Work out the finished part from the listing and answer in its coordinate system (mm). Face numbers are marked on the shaded views. A direction names the side the tool comes from. Give positions to 0.01 mm unless a question says otherwise; leave off trailing zeros. Loops run counter-clockwise (first coordinate to the right, second up) from the corner with the lowest first, then second, coordinate; pieces in that order, holes last. Notation, with made-up numbers: M -27,-36 L -8,-36 A23 ccw -8,-9 Z; hole C 64.5,23.25 d2. An arc over 180 degrees is marked long. Use a Markdown table: item, result.
```python
from build123d import *

# Parameters (mm, degrees)
F1_DEPTH = 25
F2_R     = 9.5
F3_DEPTH = 5
F4_R     = 2
F5_DEPTH = 30.001
F6_R     = 4.5
F7_DEPTH = 7
F8_R     = 1.75
F9_DEPTH = 25.001


with BuildPart() as f1:
    # F0 (on Top) → F1 (new body)
    with BuildSketch(Plane.XY):
        Polygon((-12.365591, 25), (-12.365591, 0), (12.634409, 0), (12.634409, 25), (9.434409, 25), (9.434409, 5), (-9.165591, 5), (-9.165591, 25), align=None)
    extrude(amount=F1_DEPTH)

    # F2 (on face) → F3 (join)
    with BuildSketch(Plane.XZ):
        with Locations((0.134409, 12.5)):
            Circle(F2_R)
    extrude(amount=F3_DEPTH)

    # F4 (on face) → F5 (cut, through all)
    with BuildSketch(Plane.XZ.offset(5)):
        with Locations((0.134409, 12.5)):
            Circle(F4_R)
    extrude(amount=-F5_DEPTH, mode=Mode.SUBTRACT)

    # F6 (on face) → F7 (cut)
    with BuildSketch(Plane(origin=(0, 5, 0), x_dir=(-1, 0, 0), z_dir=(0, 1, 0))):
        with Locations((-0.134409, 12.5)):
            Circle(F6_R)
    extrude(amount=-F7_DEPTH, mode=Mode.SUBTRACT)

    # F8 (on face) → F9 (cut, through all)
    with BuildSketch(Plane(origin=(-12.365591, 0, 0), x_dir=(0, -1, 0), z_dir=(-1, 0, 0))):
        with Locations((-17, 6)):
            Circle(F8_R)
        with Locations((-17, 19)):
            Circle(F8_R)
    extrude(amount=-F9_DEPTH, mode=Mode.SUBTRACT)


solid = f1.part
```
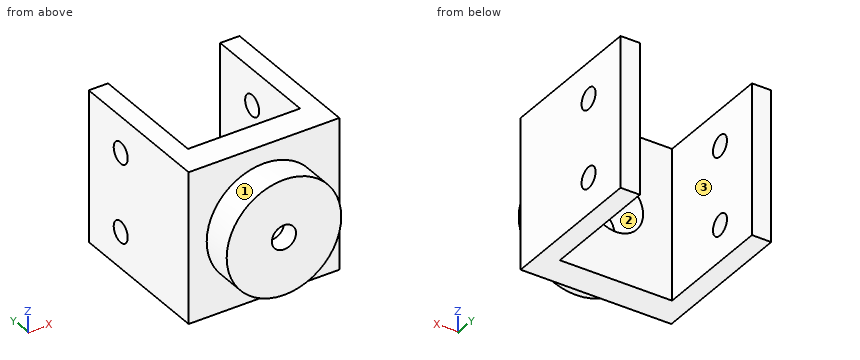
(1) Given P1, Ø2.5, axis at x = 1, z = 10.5, coming from the +Y side; P2, Ø1.5, axis at x = 6.5, z = 16.5, coming from the +Y side, each flat-ended and moving along its own axis, determine where each tip first touches the part or whether it passes through.
Entries:
| item | result |
|---|---|
| P1 | stops at y = -2 |
| P2 | stops at y = 5 |
(2) A cutting plane is placed at B-B (z = 12.5). Write down the section's boundary in (x, y).
Entries:
| item | result |
|---|---|
| outline | M -12.37,0 L -9.37,0 L -9.37,-5 L -1.87,-5 L -1.87,-2 L -4.37,-2 L -4.37,5 L -9.17,5 L -9.17,25 L -12.37,25 Z; M 2.13,-5 L 9.63,-5 L 9.63,0 L 12.63,0 L 12.63,25 L 9.43,25 L 9.43,5 L 4.63,5 L 4.63,-2 L 2.13,-2 Z |
(3) A cutting plane is placed at A-A (y = 17). Write down the section's boundary in (x, z), and give its area (3 significant figures).
Entries:
| item | result |
|---|---|
| outline | M -12.37,0 L -9.17,0 L -9.17,4.25 L -12.37,4.25 Z; M -12.37,7.75 L -9.17,7.75 L -9.17,17.25 L -12.37,17.25 Z; M -12.37,20.75 L -9.17,20.75 L -9.17,25 L -12.37,25 Z; M 9.43,0 L 12.63,0 L 12.63,4.25 L 9.43,4.25 Z; M 9.43,7.75 L 12.63,7.75 L 12.63,17.25 L 9.43,17.25 Z; M 9.43,20.75 L 12.63,20.75 L 12.63,25 L 9.43,25 Z |
| area | 115 mm² |
(4) Consider probe 1 along Z at (x, y) = (-11.15, 17); probe 2 along X at (y, z) = (5.5, 19); probe 3 along Y at (x, z) = (-6, 12). Determine where each line is inside the solid, lowest interval first. Write a range as [from, to].
Entries:
| item | result |
|---|---|
| probe 1 | z = [0, 4.25], [7.75, 17.25], [20.75, 25] |
| probe 2 | x = [-12.37, -9.17], [9.43, 12.63] |
| probe 3 | y = [-5, 5] |
(5) A cutting plane is placed at C-C (y = 5.75). Write down the section's boundary in (x, z), and give its area (3 significant figures).
Entries:
| item | result |
|---|---|
| outline | M -12.37,0 L -9.17,0 L -9.17,25 L -12.37,25 Z; M 9.43,0 L 12.63,0 L 12.63,25 L 9.43,25 Z |
| area | 160 mm² |
(6) Which of the six approach directions +Z, -Z, +X, -X, +Y, -Y give full straight-line access (tool end or side, diameter ignored) to the marked faces 1, 2 and 3?
Entries:
| item | result |
|---|---|
| face 1 | -Y |
| face 2 | +Y |
| face 3 | +Z, -Z, +Y |
(7) A cutting plane is placed at D-D (x = -0.5). Write down the section's boundary in (y, z).
Entries:
| item | result |
|---|---|
| outline | M -5,3.02 L 0,3.02 L 0,0 L 5,0 L 5,8.04 L -2,8.04 L -2,10.6 L -5,10.6 Z; M -5,14.4 L -2,14.4 L -2,16.96 L 5,16.96 L 5,25 L 0,25 L 0,21.98 L -5,21.98 Z |
